from build123d import *

# Parameters (mm, degrees)
SKETCH1_W           = 85.5
SKETCH1_H           = 39
BOSS_EXTRUDE1_DEPTH = 3
SKETCH2_W           = 85.5
SKETCH2_H           = 39
SKETCH2_W_2         = 82
SKETCH2_H_2         = 35.5
BOSS_EXTRUDE2_DEPTH = 5
SKETCH3_W           = 1.75
SKETCH3_H           = 15
BOSS_EXTRUDE3_DEPTH = 23.8
BOSS_EXTRUDE4_DEPTH = 15


with BuildPart() as part:
    # Sketch1 → Boss-Extrude1 (new body)
    with BuildSketch(Plane(origin=(0, 0, 0), x_dir=(1, 0, 0), z_dir=(0, 1, 0))):
        with Locations((42.75, 19.5)):
            Rectangle(SKETCH1_W, SKETCH1_H)
    extrude(amount=BOSS_EXTRUDE1_DEPTH)

    # Sketch2 → Boss-Extrude2 (add)
    with BuildSketch(Plane(origin=(0, 3, 0), x_dir=(1, 0, 0), z_dir=(0, 1, 0))):
        with Locations((42.75, 19.5)):
            Rectangle(SKETCH2_W, SKETCH2_H)
        with Locations((42.75, 19.5)):
            Rectangle(SKETCH2_W_2, SKETCH2_H_2, mode=Mode.SUBTRACT)
    extrude(amount=BOSS_EXTRUDE2_DEPTH)

    # Sketch3 → Boss-Extrude3 (add)
    with BuildSketch(Plane(origin=(0, 8, 0), x_dir=(1, 0, 0), z_dir=(0, 1, 0))):
        with Locations((0.875, 19.5)):
            Rectangle(SKETCH3_W, SKETCH3_H)
        with Locations((84.625, 19.5)):
            Rectangle(SKETCH3_W, SKETCH3_H)
    extrude(amount=BOSS_EXTRUDE3_DEPTH)

    # Sketch4 → Boss-Extrude4 (add)
    with BuildSketch(Plane.XY.offset(-12)):
        with BuildLine():
            Line((1.75, 31.8), (3.75, 31.8))
            Line((3.75, 31.8), (1.75, 37.294954839))
            ThreePointArc((1.75, 37.294954839), (0.745538584, 37.874880908), (0, 36.986382623))
            Line((0, 36.986382623), (0, 31.8))
            Line((0, 31.8), (1.75, 31.8))
        make_face()
        with BuildLine():
            Line((83.75, 31.8), (85.5, 31.8))
            Line((85.5, 31.8), (85.5, 36.986382623))
            ThreePointArc((85.5, 36.986382623), (84.754461416, 37.874880908), (83.75, 37.294954839))
            Line((83.75, 37.294954839), (81.75, 31.8))
            Line((81.75, 31.8), (83.75, 31.8))
        make_face()
    extrude(amount=-BOSS_EXTRUDE4_DEPTH)


solid = part.part
Can you work these out from the model? Positions are in its coordinate system, mm. A direction names the side the tool comes from. Give positions to 0.01 mm unless a question says otherwise; leave off trailing zeros. Loops run counter-clockwise (first coordinate to the right, second up) from the corner with the lowest first, then second, coordinate; pieces in that order, holes last. Notation, with made-up numbers: (41.5, 4) - (56.5, 4) arc R27 ccw to (56.5, 27) - close; hole circle Ø3 at (63, -4). An arc over 180 degrees is marked (long way). One line per item, written item: value.
(1) On a 3-axis mill with a long thin cutter (end or side, diameter ignored), from which of +Z, -Z, +X, -X, +Y, -Y can I reach the whole of each face in a straight line? I mean faces 4 (the face through (83.75, 14, -19)), 5 (the face through (42, 5, -37.25)), 6 (the face through (36.22, 8, -1.58)), 7 (the face through (82.764, 34.586, -19.395)), 8 (the face through (36.2, 8, -37.5)). Say none if no direction works.
Verdict:
face 4: none
face 5: +Y
face 6: +Z, +X, -X, +Y
face 7: +Z, -Z, +Y
face 8: -Z, +X, -X, +Y
(2) If we section it at A-A, the plane y = 4.5: List the corners of the cut face in (x, z) for me, plus the area to 4 significant figures.
Verdict:
outline: (0, -39) - (85.5, -39) - (85.5, 0) - (0, 0) - close; hole (1.75, -37.25) - (83.75, -37.25) - (83.75, -1.75) - (1.75, -1.75) - close
area: 423.5 mm^2
(3) If we section it at B-B, the plane y = 17: List the corners of the cut face in (x, z) for me, plus the area to 3 significant figures.
Verdict:
outline: (0, -27) - (1.75, -27) - (1.75, -12) - (0, -12) - close; (83.75, -27) - (85.5, -27) - (85.5, -12) - (83.75, -12) - close
area: 52.5 mm^2
(4) I need wall thicknesses on line 1 along X through (y, z) = (5, -26.5); line 2 along Z through (x, y) = (71, 4); line 3 along Y through (x, z) = (7, -11). Which ranges of each line are inside material? Lowest first, please.
Verdict:
line 1: 0 to 1.75, 83.75 to 85.5
line 2: -39 to -37.25, -1.75 to 0
line 3: 0 to 3
(5) If we mould it in two halves opening along Z, with no side actions, what happens to faces 1 (the face through (2.764, 34.509, -19.395)), 2 (the face through (1, 23, -27)), 3 (the face through (1.75, 14, -19))? For each: released by +Z, released by -Z, zero draft, split by the parting line, or undercut.
Verdict:
face 1: zero draft
face 2: released by -Z
face 3: undercut
(6) If we section it at D-D, the plane x = 6.5: List the corners of the cut face in (y, z) for me, plus the area to 4 significant figures.
Verdict:
outline: (0, -39) - (8, -39) - (8, -37.25) - (3, -37.25) - (3, -1.75) - (8, -1.75) - (8, 0) - (0, 0) - close
area: 134.5 mm^2
(7) If we section it at C-C, the plane z = -6: List the corners of the cut face in (x, y) for me.
Verdict:
outline: (0, 0) - (85.5, 0) - (85.5, 8) - (83.75, 8) - (83.75, 3) - (1.75, 3) - (1.75, 8) - (0, 8) - close
(8) I'm going to push flat-ended pins straight in: pin 1 (13 mm diameter, centred on x = 27, z = -35, fed in from +Y); pin 2 (18 mm diameter, centred on x = 53.5, z = -12, fed in from +Y); pin 3 (1.1 mm diameter, centred on x = 2, y = 29, fed in from -Z). Where does each tip first touch, or does it pass through?
Verdict:
pin 1: y = 8
pin 2: y = 3
pin 3: z = -27
